The model under review builds one solid part; all positions refer to its coordinate system, in mm. Give positions to 0.01 mm unless a question says otherwise; leave off trailing zeros. Loops run counter-clockwise (first coordinate to the right, second up) from the corner with the lowest first, then second, coordinate; pieces in that order, holes last. Notation, with made-up numbers: M -19,42.25 L -8,42.25 A27 cw -8,79.25 Z; hole C 29,-33 d3. An arc over 180 degrees is marked long. Return JSON: item names as keys, results as strings.
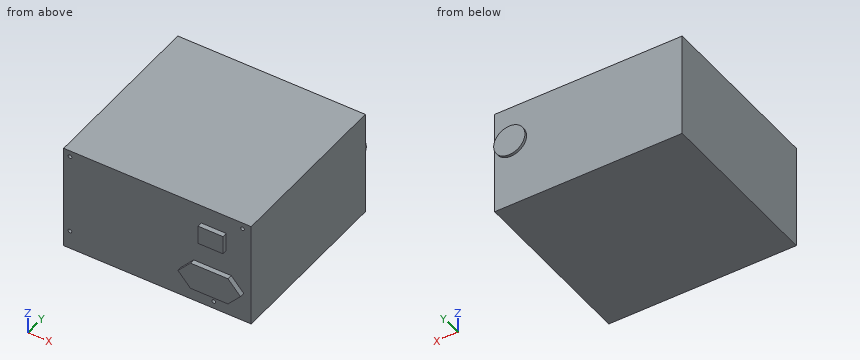
```python
from build123d import *

# Parameters (mm, degrees)
SCHIZZO1_W                   = 150
SCHIZZO1_H                   = 140
ESTRUSIONE_ESTRUSIONE1_DEPTH = 85
SCHIZZO2_W                   = 20
SCHIZZO2_H                   = 15
SCHIZZO2_W_2                 = 30
SCHIZZO2_H_2                 = 11
ESTRUSIONE_ESTRUSIONE2_DEPTH = 4
SCHIZZO3_R                   = 1.5
TAGLIO_ESTRUSIONE1_DEPTH     = 10
SCHIZZO4_R                   = 12.5
ESTRUSIONE_ESTRUSIONE3_DEPTH = 2


with BuildPart() as part:
    # Schizzo1 → Estrusione-Estrusione1 (new body)
    with BuildSketch(Plane.XY):
        with Locations((75, 70)):
            Rectangle(SCHIZZO1_W, SCHIZZO1_H)
    extrude(amount=ESTRUSIONE_ESTRUSIONE1_DEPTH)

    # Schizzo2 → Estrusione-Estrusione2 (add)
    with BuildSketch(Plane.XZ):
        with Locations((120, 62.5)):
            Rectangle(SCHIZZO2_W, SCHIZZO2_H)
        Polygon((104, 35), (94, 24), (104, 24), align=None)
        Polygon((94, 24), (104, 13), (104, 24), align=None)
        with Locations((119, 29.5)):
            Rectangle(SCHIZZO2_W_2, SCHIZZO2_H_2)
        with Locations((119, 18.5)):
            Rectangle(SCHIZZO2_W_2, SCHIZZO2_H_2)
        Polygon((134, 35), (134, 24), (144, 24), align=None)
        Polygon((134, 24), (134, 13), (144, 24), align=None)
    extrude(amount=ESTRUSIONE_ESTRUSIONE2_DEPTH)

    # Schizzo3 → Taglio-Estrusione1 (cut)
    with BuildSketch(Plane.XZ):
        with Locations(Location((5, 80, 0), (0, 0, 270))):
            Circle(SCHIZZO3_R)
        with Locations(Location((5, 15, 0), (0, 0, 270))):
            Circle(SCHIZZO3_R)
        with Locations(Location((120, 6, 0), (0, 0, 270))):
            Circle(SCHIZZO3_R)
        with Locations(Location((143, 80, 0), (0, 0, 270))):
            Circle(SCHIZZO3_R)
    extrude(amount=-TAGLIO_ESTRUSIONE1_DEPTH, mode=Mode.SUBTRACT)

    # Schizzo4 → Estrusione-Estrusione3 (add)
    with BuildSketch(Plane(origin=(0, 140, 0), x_dir=(1, 0, 0), z_dir=(0, 1, 0))):
        with Locations(Location((137, -55, 0), (0, 0, 90))):
            Circle(SCHIZZO4_R)
    extrude(amount=ESTRUSIONE_ESTRUSIONE3_DEPTH)


solid = part.part
```
1) Wall thickness on L1, parallel to X at y = 3, z = 80; L2, parallel to Z at x = 143, y = 6; L3, parallel to X at y = 5.5, z = 6: over which ranges is each line inside the solid? List them lowest first. Write a range as from..to.
From the geometry:
{"L1": "0..3.5, 6.5..141.5, 144.5..150", "L2": "0..78.5, 81.5..85", "L3": "0..118.5, 121.5..150"}
2) Consider section A-A on x = 101. Write out the cut boundary in (y, z), then the cut area to 3 significant figures.
From the geometry:
{"outline": "M -4,16.3 L 0,16.3 L 0,0 L 140,0 L 140,85 L 0,85 L 0,31.7 L -4,31.7 Z", "area": "12,000 mm²"}
3) Consider section C-C on x = 137. Write out the cut boundary in (y, z), then the cut area to 3 significant figures.
From the geometry:
{"outline": "M -4,16.3 L 0,16.3 L 0,0 L 140,0 L 140,42.5 L 142,42.5 L 142,67.5 L 140,67.5 L 140,85 L 0,85 L 0,31.7 L -4,31.7 Z", "area": "12,000 mm²"}
4) Consider section B-B on z = 39. Write out the cut boundary in (x, y).
From the geometry:
{"outline": "M 0,0 L 150,0 L 150,140 L 0,140 Z"}
5) Consider section D-D on x = 45. Write out the cut boundary in (y, z), then the cut area to 3 significant figures.
From the geometry:
{"outline": "M 0,0 L 140,0 L 140,85 L 0,85 Z", "area": "11,900 mm²"}
6) Insertion check: pin 1 (3 mm diameter, centred on y = -3, z = 64, fed in from +X); pin 2 (2 mm diameter, centred on x = 115.5, y = -2, fed in from -Z); pin 3 (3 mm diameter, centred on x = 112, y = -2, fed in from +Z); pin 4 (4 mm diameter, centred on x = 50, y = 31, fed in from -Z). Each pin has a flat end and moves straight along its axis. Give the tip position at first contact, or say it passes through.
From the geometry:
{"pin 1": "x = 130", "pin 2": "z = 13", "pin 3": "z = 70", "pin 4": "z = 0"}
